```python
from build123d import *

# Parameters (mm, degrees)
SKETCH1_W           = 224
SKETCH1_H           = 15
BOSS_EXTRUDE1_DEPTH = 2.8
SKETCH2_W           = 199
SKETCH2_H           = 2
BOSS_EXTRUDE2_DEPTH = 2
SKETCH3_R           = 1.6
CUT_EXTRUDE1_DEPTH  = 113.285751545
FILLET1_R           = 10
FILLET2_R           = 1.5


with BuildPart() as part:
    # Sketch1 → Boss-Extrude1 (new body)
    with BuildSketch(Plane(origin=(0, 0, 0), x_dir=(1, 0, 0), z_dir=(0, 1, 0))):
        Rectangle(SKETCH1_W, SKETCH1_H)
    extrude(amount=BOSS_EXTRUDE1_DEPTH)

    # Sketch2 → Boss-Extrude2 (add)
    with BuildSketch(Plane(origin=(0, 2.8, 0), x_dir=(1, 0, 0), z_dir=(0, 1, 0))):
        with Locations((-12.5, 0)):
            Rectangle(SKETCH2_W, SKETCH2_H)
    extrude(amount=BOSS_EXTRUDE2_DEPTH)

    # Sketch3 → Cut-Extrude1 (cut, through all)
    with BuildSketch(Plane(origin=(0, 2.8, 0), x_dir=(1, 0, 0), z_dir=(0, 1, 0))):
        with Locations(Location((94, 0, 0), (0, 0, 270))):
            Circle(SKETCH3_R)
    extrude(amount=-CUT_EXTRUDE1_DEPTH, mode=Mode.SUBTRACT)

    # Fillet1
    # the kernel refuses this fillet: 10 mm, written as the material it adds along each edge
    with BuildSketch(Plane(origin=(-112, 2.8, -1), x_dir=(0, 0, -1), z_dir=(1, 0, 0)), Plane(origin=(87, 2.8, 1), x_dir=(0, 0, 1), z_dir=(-1, 0, 0))) as fillet1_piece_1:
        with BuildLine():
            CenterArc((6, 10), FILLET1_R, 233.130102354, 36.869897646)
            Line((0, 2), (0, 0))
            Line((0, 0), (6, 0))
        make_face()
    extrude(amount=199)

    # Fillet2
    # the kernel refuses this fillet: 1.5 mm, written as the material it takes off along each edge
    with BuildSketch(Plane(origin=(112, 0, -11.25), x_dir=(0, 1, 0), z_dir=(0, 0, 1))) as fillet2_piece_1:
        with BuildLine():
            CenterArc((FILLET2_R, FILLET2_R), FILLET2_R, 180, 90)
            Line((0, FILLET2_R), (0, 0))
            Line((0, 0), (FILLET2_R, 0))
        make_face()
    extrude(amount=22.5, mode=Mode.SUBTRACT)
    with BuildSketch(Plane(origin=(112, 2.8, -11.25), x_dir=(0, -1, 0), z_dir=(0, 0, 1))) as fillet2_piece_2:
        with BuildLine():
            CenterArc((FILLET2_R, -FILLET2_R), FILLET2_R, 90, 90)
            Line((0, -FILLET2_R), (0, 0))
            Line((0, 0), (FILLET2_R, 0))
        make_face()
    extrude(amount=22.5, mode=Mode.SUBTRACT)


solid = part.part
```
Source: CAD feature listing. Evaluate the final solid. Frame: model axes, mm. A direction names the side the tool comes from. Coordinates: 2 decimals unless noted, no trailing zeros. Loops run counter-clockwise (first coordinate to the right, second up) from the corner with the lowest first, then second, coordinate; pieces in that order, holes last. Notation, with made-up numbers: (59.25, -2.75) -> (86.25, -2.75) arc R23 cw to (86.25, 18.25) -> close; hole circle Ø2 at (36, 55). An arc over 180 degrees is marked (long way). One line per item, written item: value. Start each with the question number.
Q1. Section query A-A, the plane x = -49. Return the cut outline in (y, z).
Q2. Section query B-B, the plane z = -5. Return the cut outline in (x, y).
Q3. Section query C-C, the plane y = 3.8. Return the cut outline in (x, z), and give its area (3 significant figures).
Q4. Section query D-D, the plane z = 4. Return the cut outline in (x, y), and give its area (3 significant figures).
Q5. Set-up query: faces 1 (the face through (-2, 0, 0)), 2 (the face through (56.4, 2.8, 7.2)). Return all of +Z, -Z, +X, -X, +Y, -Y with unobstructed straight access to the full face (end or side cutting, diameter ignored); none if empty.
Q6. Line query: line 1 along Z through (x, y) = (94, 2.15); line 2 along X through (y, z) = (1.2, 0); line 3 along X through (y, z) = (0.8, 0). Output: solid intervals per line, ascending.
Results:
1. outline: (0, -7.5) -> (2.8, -7.5) -> (2.8, -7) arc R10 cw to (4.8, -1) -> (4.8, 1) arc R10 cw to (2.8, 7) -> (2.8, 7.5) -> (0, 7.5) -> close
2. outline: (-112, 0) -> (110.5, 0) arc R1.5 ccw to (112, 1.4) arc R1.5 ccw to (110.5, 2.8) -> (87, 2.8) -> (87, 3) -> (-112, 3) -> close
3. outline: (-112, -2.64) -> (87, -2.64) -> (87, 2.64) -> (-112, 2.64) -> close
3. area: 1,050 mm^2
4. outline: (-112, 0) -> (110.5, 0) arc R1.5 ccw to (112, 1.4) arc R1.5 ccw to (110.5, 2.8) -> (87, 2.8) -> (87, 3.26) -> (-112, 3.26) -> close
4. area: 718 mm^2
5. face 1: +Z, -Z, +X, -X, -Y
5. face 2: +X, +Y
6. line 1: -7.5 to -1.6, 1.6 to 7.5
6. line 2: -112 to 92.4, 95.6 to 111.97
6. line 3: -112 to 92.4, 95.6 to 111.83
